```python
from build123d import *

# Parameters (mm, degrees)
SKETCH3_R           = 0.21
BOSS_EXTRUDE1_DEPTH = 0.2
CIRPATTERN1_COUNT   = 6


with BuildPart() as part:
    # Sketch2 → Revolve1 (revolve)
    with BuildSketch(Plane.XY, mode=Mode.PRIVATE) as revolve1_sk:
        Polygon((-1.81, 2.68), (-1.81, 4.68), (-1.56, 4.68), (-1.56, 6.78), (-1.3, 6.78), (-1.3, 9.32), (-2.9, 9.32), (-2.9, 6.38), (-3.24, 6.38), (-3.24, 6.18), (-3.64, 6.18), (-3.64, 6.08), (-8.8, 6.08), (-8.8, 6.18), (-9.4, 6.18), (-9.4, 6.38), (-11.1, 6.38), (-11.4, 6.08), (-11.4, 4.03), (-11.1, 3.73), (-9.4, 3.73), (-2.54, 4.34), (-2.54, 4.289146726), (-2.61, 4.289146726), (-2.61, 4.03), (-2.5, 4.03), (-2.5, 2.68), align=None)
    revolve(revolve1_sk.sketch.rotate(Axis((0, 0, 0), (0, 1, 0)), 270), axis=Axis((0, 0, 0), (0, 1, 0)))

    # Sketch3 → Boss-Extrude1 (add)
    with BuildSketch(Plane(origin=(0, 6.18, 0), x_dir=(1, 0, 0), z_dir=(0, 1, 0))):
        with Locations(Location((0, 9.1, 0), (0, 0, 90))):
            Circle(SKETCH3_R)
    boss_extrude1 = extrude(amount=BOSS_EXTRUDE1_DEPTH)

    # CirPattern1: Boss-Extrude1 ×6 about axis
    cirpattern1_axis = Axis((0, 0, 0), (0, 1, 0))
    for i in range(1, CIRPATTERN1_COUNT):
        add(boss_extrude1.rotate(cirpattern1_axis, i * 360 / CIRPATTERN1_COUNT))


solid = part.part
```
Input: part model. Units: mm. Frame: model coordinates. A direction names the side the tool comes from. Give positions to 0.01 mm unless a question says otherwise; leave off trailing zeros. Order: outer loops, then holes, each group sorted by start corner. A loop starts at its lowest first (then second) coordinate and runs counter-clockwise, first axis right, second up. Notation, with made-up numbers: M -10,60 L 21,60 A20 ccw 21,87 Z; hole C 35,-34.75 d2. An arc over 180 degrees is marked long. One line per question, with ' | ' between items. Start each with the question number.
1. First-contact query: pin 1 Ø1.5 at (x, y) = (-3, 4.5) entering from +Z; pin 2 Ø0.5 at (x, z) = (-8, 4.5) entering from +Y; pin 3 Ø3 at (y, z) = (6.5, -8) entering from -X. Flat tips, straight axial feed; report the tip coordinate or a pass-through.
2. Material intervals for probe 1 along Y at (x, z) = (-7.5, -7.5); probe 2 along Z at (x, y) = (7.25, 4.25); probe 3 along Y at (x, z) = (5.25, 7.75), sorted ascending. Write a range as [from, to].
3. Section query A-A (y = 8.5). Return the cut outline in (x, z), and give its area (3 significant figures).
4. Access query for faces 1 (the face through (2.44, 3.35, 0.54)), 2 (the face through (7, 5, 9)), 3 (the face through (0, 6.08, 4)). Directions: +Z, -Z, +X, -X, +Y, -Y. A direction counts if a zero-diameter tool reaches every point of the face in a straight line with its end or side. Return the directions, or none.
5. Section query B-B (y = 5). Return the cut outline in (x, z).
Here are the results:
1) pin 1: z = 11.18 | pin 2: y = 6.38 | pin 3: x = -9.32
2) probe 1: [3.73, 6.38] | probe 2: [-8.8, 8.8] | probe 3: [3.73, 6.18]
3) outline: C 0,0 d5.8; hole C 0,0 d2.6 | area: 21.1 mm²
4) face 1: -Y | face 2: +Y, -Y | face 3: +Y
5) outline: C 0,0 d22.8; hole C 0,0 d3.12
